```python
from build123d import *

# Parameters (mm, degrees)
F1_DEPTH = 9.525
F2_DEPTH = 6.35
F3_R     = 6.35
F4_DEPTH = 9.526
F5_SIZE  = 6.35


with BuildPart() as f1:
    # F0 (on Front) → F1 (new body)
    with BuildSketch(Plane.XZ):
        with BuildLine():
            Line((-44.45, 63.5), (-44.45, 0))
            Line((-44.45, 0), (44.45, 0))
            Line((44.45, 0), (44.45, 63.5))
            ThreePointArc((44.45, 63.5), (23.58629, 82.8043), (15.875, 110.16278))
            Line((15.875, 110.16278), (15.875, 177.8))
            Line((15.875, 177.8), (-15.875, 177.8))
            Line((-15.875, 177.8), (-15.875, 110.16278))
            ThreePointArc((-15.875, 110.16278), (-23.58629, 82.8043), (-44.45, 63.5))
        make_face()
    extrude(amount=-F1_DEPTH)

    # F0 (on Front) → F2 (join)
    with BuildSketch(Plane.XZ):
        with BuildLine():
            Line((-44.45, 63.5), (-44.45, 0))
            Line((-44.45, 0), (44.45, 0))
            Line((44.45, 0), (44.45, 63.5))
            ThreePointArc((44.45, 63.5), (23.58629, 82.8043), (15.875, 110.16278))
            Line((15.875, 110.16278), (15.875, 177.8))
            Line((15.875, 177.8), (-15.875, 177.8))
            Line((-15.875, 177.8), (-15.875, 110.16278))
            ThreePointArc((-15.875, 110.16278), (-23.58629, 82.8043), (-44.45, 63.5))
        make_face()
    extrude(amount=-F2_DEPTH)

    # F3 (on face) → F4 (cut, through all)
    with BuildSketch(Plane.XZ):
        with Locations((0, 158.75)):
            Circle(F3_R)
    extrude(amount=-F4_DEPTH, mode=Mode.SUBTRACT)

    # F5
    f5_edges = [f1.edges().sort_by_distance(p)[0] for p in [
        (15.875, 4.7625, 177.8),
        (-15.875, 4.7625, 177.8),
    ]]
    chamfer(f5_edges, length=F5_SIZE)


solid = f1.part
```
Verification items for the finished model (mm, model axes). A direction names the side the tool comes from. Coordinates: 2 decimals unless noted, no trailing zeros. Order: outer loops, then holes, each group sorted by start corner. A loop starts at its lowest first (then second) coordinate and runs counter-clockwise, first axis right, second up. Notation, with made-up numbers: (-16, 14) -> (34, 14) arc R24 cw to (34, 53) -> close; hole circle Ø1 at (37, 3). An arc over 180 degrees is marked (long way). Put each result on its own line as item: value. Start each with the question number.
1) Cross-section at D-D (z = 122.5). Enter the section's corners in (x, y) (3 decimals), plus the area to 3 significant figures.
2) Cross-section at C-C (z = 158.75). Enter the section's corners in (x, y) (3 decimals), plus the area to 3 significant figures.
3) Release check for a two-part mould opening along Z. For faces 4 (the flat face through (12.744, 4.829, 174.581)), 5 (the flat face through (-1, 9.525, 70)), 6 (the cylindrical face through (-0.827, 4.696, 165.046)), 7 (the flat face through (-1, 5, 0)) record: pulls with the +Z half, pulls with the -Z half, needs draft (parallel to the pull), parting line crosses it, or undercut.
4) Material ranges on L1, parallel to Z at x = 0, y = 2.75; L2, parallel to X at y = 3.75, z = 151 (3 decimals); L3, parallel to Z at x = -29.5, y = 4, recorded low to high.
5) Go/stop test with flat-tipped pins: pin 1 (10 mm diameter, centred on x = -24.5, z = 148, fed in from -Y); pin 2 (1.5 mm diameter, centred on y = 8, z = 126.5, fed in from +X) (3 decimals); pin 3 (5 mm diameter, centred on y = 6.5, z = 130, fed in from -X) (3 decimals); pin 4 (2 mm diameter, centred on y = 6.5, z = 79.5, fed in from +X). Record where each tip stops, or that it passes through.
6) Tool access check on faces 1 (the flat face through (0, 5, 177.8)), 2 (the flat face through (-15.875, 5, 141)), 3 (the flat face through (15.875, 5, 140)). Record the directions out of +Z, -Z, +X, -X, +Y, -Y that give a thin tool (end or side, any length) a straight path to the whole face; none if there is none.
7) Cross-section at A-A (x = 0). Enter the section's corners in (y, z) (3 decimals).
Geometry check:
1. outline: (-15.875, 0) -> (15.875, 0) -> (15.875, 9.525) -> (-15.875, 9.525) -> close
1. area: 302 mm^2
2. outline: (-15.875, 0) -> (-6.35, 0) -> (-6.35, 9.525) -> (-15.875, 9.525) -> close; (6.35, 0) -> (15.875, 0) -> (15.875, 9.525) -> (6.35, 9.525) -> close
2. area: 181 mm^2
3. face 4: pulls with the +Z half
3. face 5: needs draft
3. face 6: undercut
3. face 7: pulls with the -Z half
4. L1: z = 0 to 152.4, 165.1 to 177.8
4. L2: x = -15.875 to 15.875
4. L3: z = 0 to 74.92
5. pin 1: passes through
5. pin 2: stops at x = 15.875
5. pin 3: stops at x = -15.875
5. pin 4: stops at x = 26.53
6. face 1: +Z, +X, -X, +Y, -Y
6. face 2: +Z, -X, +Y, -Y
6. face 3: +Z, +X, +Y, -Y
7. outline: (0, 0) -> (9.525, 0) -> (9.525, 152.4) -> (0, 152.4) -> close; (0, 165.1) -> (9.525, 165.1) -> (9.525, 177.8) -> (0, 177.8) -> close
